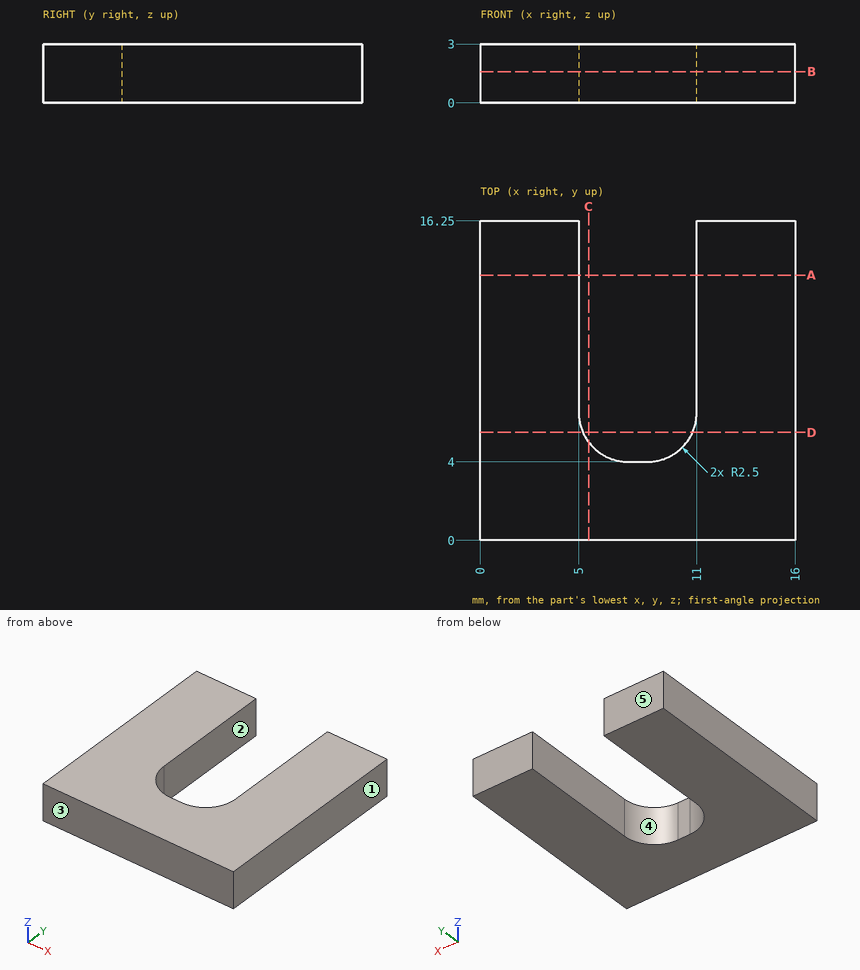
Input: dimensioned drawing with shaded views. Units: mm. Origin: part minimum x, y, z. A direction names the side the tool comes from. Coordinates: 2 decimals unless noted, no trailing zeros. Order: outer loops, then holes, each group sorted by start corner. A loop starts at its lowest first (then second) coordinate and runs counter-clockwise, first axis right, second up. Notation, with made-up numbers: M 33,-30.75 L 38,-30.75 A18 ccw 38,-26.75 Z; hole C 67.25,-9.75 d4. An arc over 180 degrees is marked long. Write each question's results on one line, items separated by ' | '. Start each with the question number.
Item 1: Set-up query: the marked faces 4 and 5. Return all of +Z, -Z, +X, -X, +Y, -Y with unobstructed straight access to the full face (end or side cutting, diameter ignored); none if empty.
Item 2: Cut plane D-D (y = 5.5). Return loops of the section in (x, z), and give its area (3 significant figures).
Item 3: Cut plane A-A (y = 13.5). Return loops of the section in (x, z), and give its area (3 significant figures).
Item 4: Cut plane B-B (z = 1.6). Return loops of the section in (x, y).
Item 5: Cut plane C-C (x = 5.5). Return loops of the section in (y, z), and give its area (3 significant figures).
Item 6: Line query: probe 1 along X at (y, z) = (8.5, 1.05); probe 2 along Y at (x, z) = (10.5, 0.35); probe 3 along X at (y, z) = (5.5, 2.2). Output: solid intervals per line, ascending.
Item 7: Draft query along X for the marked faces 1, 2 and 3. Return one class per face: pulls with the +X half, pulls with the -X half, needs draft (parallel to the pull), parting line crosses it, or undercut.
Item 8: First-contact query: pin 1 Ø1.1 at (x, z) = (8, 1.5) entering from +Y; pin 2 Ø1.5 at (x, z) = (13.5, 2.5) entering from -Y. Flat tips, straight axial feed; report the tip coordinate or a pass-through.
Checked values:
1) face 4: +Z, -Z, +Y | face 5: +Z, -Z, +X, -X, +Y
2) outline: M 0,0 L 5.21,0 L 5.21,3 L 0,3 Z; M 10.79,0 L 16,0 L 16,3 L 10.79,3 Z | area: 31.3 mm2
3) outline: M 0,0 L 5,0 L 5,3 L 0,3 Z; M 11,0 L 16,0 L 16,3 L 11,3 Z | area: 30.0 mm2
4) outline: M 0,0 L 16,0 L 16,16.25 L 11,16.25 L 11,6.5 A2.5 cw 8.5,4 L 7.5,4 A2.5 cw 5,6.5 L 5,16.25 L 0,16.25 Z
5) outline: M 0,0 L 5,0 L 5,3 L 0,3 Z | area: 15.0 mm2
6) probe 1: x = 0 to 5, 11 to 16 | probe 2: y = 0 to 5 | probe 3: x = 0 to 5.21, 10.79 to 16
7) face 1: pulls with the +X half | face 2: undercut | face 3: needs draft
8) pin 1: stops at y = 4 | pin 2: stops at y = 0
